Drawing for the job (mm, zero at the part's lowest x, y, z). A direction names the side the tool comes from. Give positions to 0.01 mm unless a question says otherwise; leave off trailing zeros. Order: outer loops, then holes, each group sorted by start corner. A loop starts at its lowest first (then second) coordinate and runs counter-clockwise, first axis right, second up. Notation, with made-up numbers: (52.5, 75.25) -> (105.5, 75.25) arc R8 ccw to (105.5, 83.25) -> close; hole circle Ø7 at (23.5, 80). An arc over 180 degrees is marked (long way). Use one line per item in the form item = value. Start each with the question number.
1) Cut at A-A, the plane x = 30. Give the cut face in (y, z) (3 decimals).
2) Probe line 1 (Y direction, x = 45, z = 38) (3 decimals); line 2 (Y direction, x = 16.5, z = 15); line 3 (Z direction, x = 21, y = 60). List the from-to ranges inside material, lowest first.
3) Cut at B-B, the plane z = 15. Give the cut face in (x, y), and give its area (3 significant figures).
4) Cut at C-C, the plane x = 53.5. Give the cut face in (y, z) (3 decimals).
5) Mould opens along X. For the marked faces 3, 4 and 5 say: pulls with the +X half, pulls with the -X half, needs draft (parallel to the pull), parting line crosses it, or undercut.
6) Tool access for the marked faces 1 and 2: list every direction of +Z, -Z, +X, -X, +Y, -Y with a clear straight run to the whole face (end or side of a thin tool).
7) Cut at D-D, the plane x = 12.5. Give the cut face in (y, z) (3 decimals).
8) Drop flat-ended pins along their axis: P1, Ø1, axis at x = 55, z = 10.5, coming from the -Y side; P2, Ø8, axis at x = 59.5, y = 19.5, coming from the -Z side; P3, Ø12, axis at x = 48, z = 16.5, coming from the +Y side. Give the stop position or say it passes through.
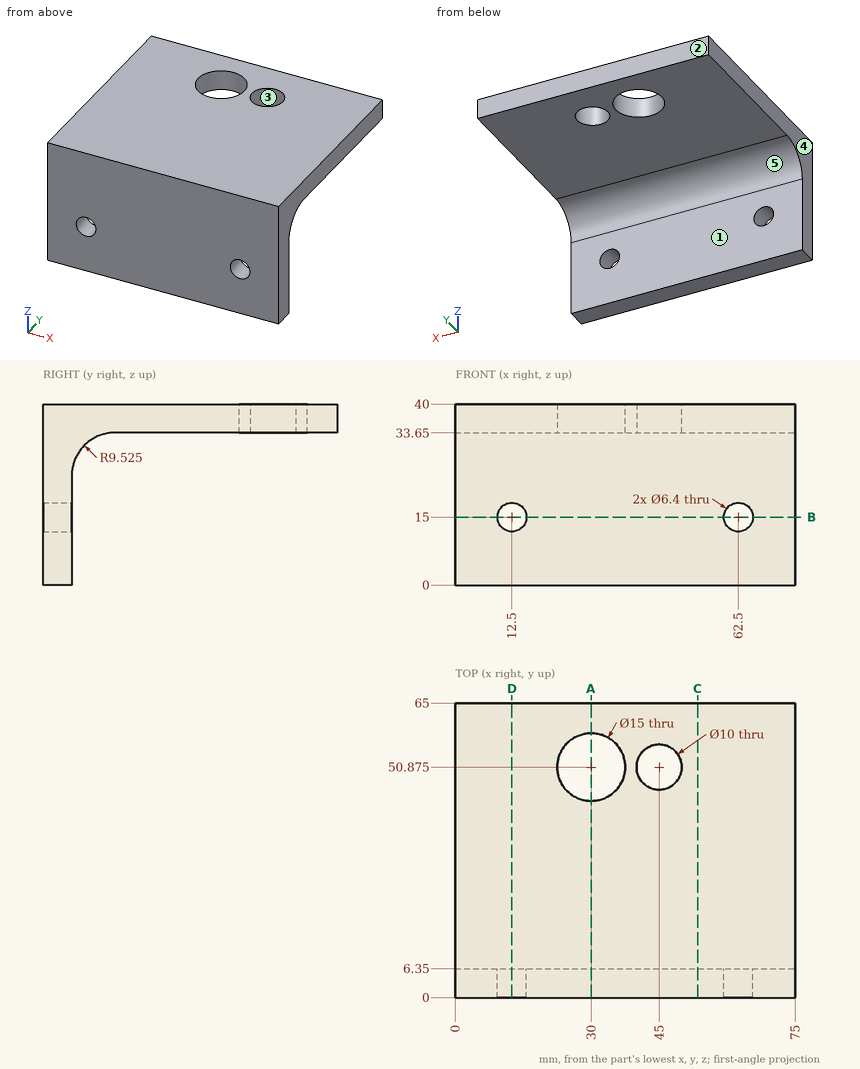
Result:
q1.outline = (0, 0) -> (6.35, 0) -> (6.35, 24.125) arc R9.525 cw to (15.875, 33.65) -> (43.375, 33.65) -> (43.375, 40) -> (0, 40) -> close; (58.375, 33.65) -> (65, 33.65) -> (65, 40) -> (58.375, 40) -> close
q2.line_1 = 0 to 45.875, 55.875 to 65
q2.line_2 = 0 to 6.35
q2.line_3 = 33.65 to 40
q3.outline = (0, 0) -> (9.3, 0) -> (9.3, 6.35) -> (0, 6.35) -> close; (15.7, 0) -> (59.3, 0) -> (59.3, 6.35) -> (15.7, 6.35) -> close; (65.7, 0) -> (75, 0) -> (75, 6.35) -> (65.7, 6.35) -> close
q3.area = 395 mm²
q4.outline = (0, 0) -> (6.35, 0) -> (6.35, 24.125) arc R9.525 cw to (15.875, 33.65) -> (65, 33.65) -> (65, 40) -> (0, 40) -> close
q5.face_3 = undercut
q5.face_4 = pulls with the -X half
q5.face_5 = needs draft
q6.face_1 = -Z, +X, -X, +Y
q6.face_2 = +Z, -Z, +X, -X, +Y
q7.outline = (0, 0) -> (6.35, 0) -> (6.35, 11.8) -> (0, 11.8) -> close; (0, 18.2) -> (6.35, 18.2) -> (6.35, 24.125) arc R9.525 cw to (15.875, 33.65) -> (65, 33.65) -> (65, 40) -> (0, 40) -> close
q8.P1 = 0
q8.P2 = 33.64
q8.P3 = 6.35
